Can you work these out from the model? Positions are in its coordinate system, mm. Face numbers are marked on the shaded views. Give positions to 0.01 mm unless a question says otherwise; leave off trailing zeros. Order: outer loops, then holes, each group sorted by start corner. A loop starts at its lowest first (then second) coordinate and runs counter-clockwise, first axis right, second up. Notation, with made-up numbers: (-22.75, -13) - (4.25, -13) arc R9 ccw to (4.25, 1) - close; hole circle Ø2 at (74, 85). An arc over 180 degrees is marked (long way). Return JSON: item names as keys, results as strings.
```python
from build123d import *
from build123d.topology import SkipClean

# Parameters (mm, degrees)
SKETCH_1_R                  = 5
SKETCH_1_R_2                = 0.6
SKETCH_1_W                  = 40
SKETCH_1_H                  = 6
EXTRUDE_1_DEPTH             = 2.5
CUT_EXTRUDE_2_DEPTH         = 46.467021015
CUT_EXTRUDE_2_DEPTH_BACK    = 46.467021015
SKETCH_1_3_R                = 2
FILLET_1_R                  = 3
EXTRUDE_START               = -1.5
EXTRUDE_2_DEPTH             = 1.5
SKETCH_2_R                  = 1.8
EXTRUDE_4_DEPTH             = 5
EXTRUDE_5_REACH             = 48.014
SKETCH_1_5_R                = 2
EXTRUDE_5_DIRECTION_2_REACH = 48.014
SKETCH_3_W                  = 2
SKETCH_3_H                  = 3
EXTRUDE_8_DEPTH             = 1.5
SKETCH_4_W                  = 0.5
SKETCH_4_H                  = 1.5
EXTRUDE_9_DEPTH             = 2


with BuildPart() as part:
    # Sketch 1 → Extrude 1 (new body)
    # profile 1 of 3: a face of its own
    with BuildSketch(Plane(origin=(0, 0, 0), x_dir=(0, 0, -1), z_dir=(1, 0, 0))):
        Circle(SKETCH_1_R)
        with Locations((0, 4.2)):
            Circle(SKETCH_1_R_2, mode=Mode.SUBTRACT)
    # profile 2 of 3: a face of its own
    with BuildSketch(Plane(origin=(0, 0, 0), x_dir=(0, 0, -1), z_dir=(1, 0, 0))):
        with Locations((40, -1)):
            Circle(SKETCH_1_R)
    # profile 3 of 3: a face of its own
    with BuildSketch(Plane(origin=(0, 0, 0), x_dir=(0, 0, -1), z_dir=(1, 0, 0))):
        with Locations((20, 0)):
            Rectangle(SKETCH_1_W, SKETCH_1_H)
    extrude(amount=EXTRUDE_1_DEPTH)

    # Sketch 1_3 → Cut-Extrude 2 (cut, two sides: drawn at the far end of the back side and taken through both)
    with BuildSketch(Plane(origin=(0, 0, 0), x_dir=(0, 0, -1), z_dir=(1, 0, 0)).offset(-CUT_EXTRUDE_2_DEPTH_BACK)):
        Circle(SKETCH_1_3_R)
        with Locations((40, -1)):
            Circle(SKETCH_1_3_R)
    extrude(amount=CUT_EXTRUDE_2_DEPTH + CUT_EXTRUDE_2_DEPTH_BACK, mode=Mode.SUBTRACT)

    # Fillet 1
    fillet_1_edges = [part.edges().sort_by_distance(p)[0] for p in [
        (1.25, -3, -35.417424305),
        (1.25, 3, -37),
        (1.25, 3, -4),
        (1.25, -3, -4),
    ]]
    fillet(fillet_1_edges, radius=FILLET_1_R)

    # Sketch 1_4 → Extrude 2 (add)
    with SkipClean():  # the faces are left unmerged after this step: merging them gives an invalid solid
        with BuildSketch(Plane(origin=(0, 0, 0), x_dir=(0, 0, -1), z_dir=(1, 0, 0)).offset(EXTRUDE_START)):
            with BuildLine():
                ThreePointArc((37, 3), (35.16534763, 0.275200556), (35.417424305, -3))
                Line((35.417424305, -3), (40, -3))
                ThreePointArc((40, -3), (38, -1), (40, 1))
                Line((40, 1), (40, 3))
                Line((40, 3), (37, 3))
            make_face()
            with BuildLine():
                Line((40, -3), (35.417424305, -3))
                ThreePointArc((35.417424305, -3), (41.021548218, -5.894531565), (45, -1))
                ThreePointArc((45, -1), (42.236067977, 3.472135955), (37, 3))
                Line((37, 3), (40, 3))
                Line((40, 3), (40, 1))
                ThreePointArc((40, 1), (41.414213562, 0.414213562), (42, -1))
                ThreePointArc((42, -1), (41.414213562, -2.414213562), (40, -3))
            make_face()
        extrude(amount=EXTRUDE_2_DEPTH)

    # Extrude 5: up to this face of the body (flat: up to its plane)
    extrude_5_end = Plane(part.part.faces().sort_by_distance((2.5, -0.21352009, -20.113168079))[0])
    # Sketch 1_5 → Extrude 5 (add, up to the picked face)
    with BuildSketch(Plane(origin=(0, 0, 0), x_dir=(0, 0, -1), z_dir=(1, 0, 0)), mode=Mode.PRIVATE) as extrude_5_sk1:
        with Locations((40, -1)):
            Circle(SKETCH_1_5_R)
    extrude_5_tool1 = split(extrude(extrude_5_sk1.sketch, amount=EXTRUDE_5_REACH, mode=Mode.PRIVATE), bisect_by=extrude_5_end, keep=Keep.BOTH, mode=Mode.PRIVATE)


with BuildPart() as body_2:
    # Sketch 2 → Extrude 4 (new body)
    with BuildSketch(Plane(origin=(2.5, 0, 0), x_dir=(0, 0, -1), z_dir=(1, 0, 0))):
        with Locations((40, -1)):
            Circle(SKETCH_2_R)
    extrude(amount=EXTRUDE_4_DEPTH)


with BuildPart() as part_1:
    add(part.part)

    add(body_2.part)  # Extrude 5 merges body 2
    add(extrude_5_tool1.solids().sort_by(Axis((0, -1, -40), (1, 0, 0)))[0])

    # Extrude 5 direction 2: up to this face of the body (flat: up to its plane)
    extrude_5_direction_2_end = Plane(part_1.part.faces().sort_by_distance((-1.5, -3.141421356, -40))[0])
    # Sketch 1_5 → Extrude 5 direction 2 (add, up to the picked face)
    with BuildSketch(Plane(origin=(0, 0, 0), x_dir=(0, 0, -1), z_dir=(1, 0, 0)), mode=Mode.PRIVATE) as extrude_5_direction_2_sk1:
        with Locations((40, -1)):
            Circle(SKETCH_1_5_R)
    extrude_5_direction_2_tool1 = split(extrude(extrude_5_direction_2_sk1.sketch, amount=-EXTRUDE_5_DIRECTION_2_REACH, mode=Mode.PRIVATE), bisect_by=extrude_5_direction_2_end, keep=Keep.BOTH, mode=Mode.PRIVATE)
    add(extrude_5_direction_2_tool1.solids().sort_by(Axis((0, -1, -40), (-1, 0, 0)))[0])

    # Sketch 3 → Extrude 8 (add)
    with BuildSketch(Plane.ZY):
        with Locations((-20, 0)):
            Rectangle(SKETCH_3_W, SKETCH_3_H)
    extrude(amount=EXTRUDE_8_DEPTH)

    # Sketch 4 → Extrude 9 (add)
    with BuildSketch(Plane(origin=(0, 0, -21), x_dir=(-1, 0, 0), z_dir=(0, 0, -1))):
        with Locations((1.25, 0.75)):
            Rectangle(SKETCH_4_W, SKETCH_4_H)
    extrude(amount=EXTRUDE_9_DEPTH)

    # Mirror 3: part across plane


with BuildPart() as part_2:
    add(part_1.part)
    add(part_1.part.mirror(Plane.ZY.offset(1.5)))


solid = part_2.part
```
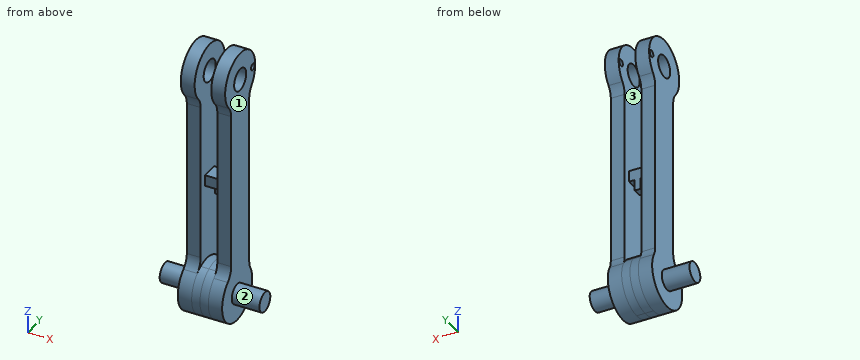
1. Thinking about a two-plate mould opening in X: for the marked faces 1, 2 and 3, which applies, +X half, -X half, draft (parallel to the pull), parting line (faces both ways), or undercut?
Checks:
{"face 1": "+X half", "face 2": "draft", "face 3": "undercut"}
2. Suppose I cut it at C-C (x = -6). List the corners of the cut face in (y, z) for me.
Checks:
{"outline": "circle Ø3.6 at (-1, -40)"}
3. If I drill on L1, parallel to Y at x = 0.65, z = 0; L2, parallel to X at y = -1.5, z = -3; L3, parallel to Z at x = -2.75, y = -0.75, over which ranges is the centre line in solid material (lowest first)? Write a range as [from, to].
Checks:
{"L1": "[-5, -2], [2, 3.6], [4.8, 5]", "L2": "[-5.5, -3], [0, 2.5]", "L3": "[-44.99, -35.01], [-21, -19]"}
4. Suppose I cut it at B-B (z = 0). List the corners of the cut face in (x, y) for me, plus the area to 3 significant figures.
Checks:
{"outline": "(-5.5, -5) - (-3, -5) - (-3, -2) - (-5.5, -2) - close; (-5.5, 2) - (-3, 2) - (-3, 3.6) - (-5.5, 3.6) - close; (-5.5, 4.8) - (-3, 4.8) - (-3, 5) - (-5.5, 5) - close; (0, -5) - (2.5, -5) - (2.5, -2) - (0, -2) - close; (0, 2) - (2.5, 2) - (2.5, 3.6) - (0, 3.6) - close; (0, 4.8) - (2.5, 4.8) - (2.5, 5) - (0, 5) - close", "area": "24.0 mm^2"}
5. For pin 1 Ø8 at (x, z) = (2.5, -6) entering from +Y; pin 2 Ø3 at (y, z) = (0, -13) entering from +X; pin 3 Ø1.5 at (x, z) = (-1.5, -21) entering from +Y; pin 4 Ø3 at (y, z) = (0, 0) entering from +X, each with a flat end and sliding along its axis, tell me the tip position at first contact or that it passes through.
Checks:
{"pin 1": "y = 4.58", "pin 2": "x = 2.5", "pin 3": "y = 1.5", "pin 4": "through"}
6. Suppose I cut it at A-A (z = -32). List the corners of the cut face in (x, y) for me, plus the area to 3 significant figures.
Checks:
{"outline": "(-5.5, -3) - (-3, -3) - (-3, 3) - (-5.5, 3) - close; (0, -3) - (2.5, -3) - (2.5, 3) - (0, 3) - close", "area": "30.0 mm^2"}
